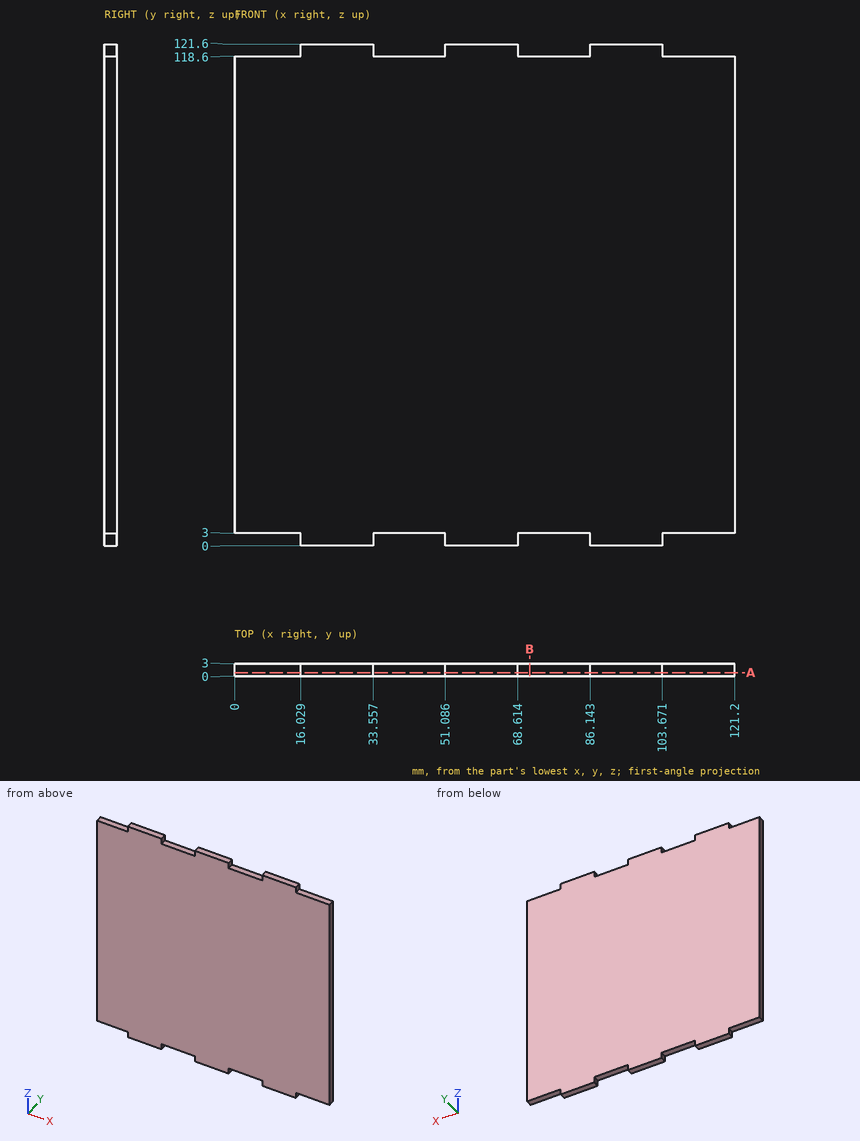
Job drawing, mm, ordinate dimensions from the low corner. One solid piece. Give positions to 0.01 mm unless a question says otherwise; leave off trailing zeros. Write each loop counter-clockwise with the first axis right and the second up, starting at its lowest first coordinate (ties: lowest second). Pieces come first, ordered by that corner, then holes. Notation, with made-up numbers: (12, 61.25) - (68, 61.25) arc R5 cw to (68, 68.25) - close; hole circle Ø2 at (88.25, -17). An arc over 180 degrees is marked (long way). Answer as CSV lines item,"result".
1. Band-saw the part on A-A (y = 0.8). Write the cut outline in (x, z) (1 decimal), and give its area (3 significant figures).
Responses:
outline,"(0, 3) - (16, 3) - (16, 0) - (33.6, 0) - (33.6, 3) - (51.1, 3) - (51.1, 0) - (68.6, 0) - (68.6, 3) - (86.1, 3) - (86.1, 0) - (103.7, 0) - (103.7, 3) - (121.2, 3) - (121.2, 118.6) - (103.7, 118.6) - (103.7, 121.6) - (86.1, 121.6) - (86.1, 118.6) - (68.6, 118.6) - (68.6, 121.6) - (51.1, 121.6) - (51.1, 118.6) - (33.6, 118.6) - (33.6, 121.6) - (16, 121.6) - (16, 118.6) - (0, 118.6) - close"
area,"14,300 mm2"
2. Drill centre line: L1, parallel to Z at x = 109.5, y = 0.6. Where is it in solid material? Low to high. Write a range as [from, to].
Responses:
L1,"z = [3, 118.6]"
3. Band-saw the part on B-B (x = 71.5). Write the cut outline in (y, z), and give its area (3 significant figures).
Responses:
outline,"(0, 3) - (3, 3) - (3, 118.6) - (0, 118.6) - close"
area,"347 mm2"
4. Pin check, flat tips, straight feed: pin 1 (1.5 mm diameter, centred on y = 2, z = 1, fed in from -X); pin 2 (0.9 mm diameter, centred on y = 1, z = 1, fed in from +X); pin 3 (12 mm diameter, centred on x = 62, z = 29.5, fed in from -Y); pin 4 (1.5 mm diameter, centred on x = 114, y = 1, fed in from -Z). Stop position of each tip, or through.
Responses:
pin 1,"stops at x = 16.03"
pin 2,"stops at x = 103.67"
pin 3,"stops at y = 0"
pin 4,"stops at z = 3"
